Design review of the part built by this model. Coordinates are the model's own, in mm. A direction names the side the tool comes from. Round coordinates to 2 decimals unless told otherwise and drop trailing zeros. Order: outer loops, then holes, each group sorted by start corner. A loop starts at its lowest first (then second) coordinate and runs counter-clockwise, first axis right, second up. Notation, with made-up numbers: (67, 18) - (116, 18) arc R20 cw to (116, 36) - close; hole circle Ø7 at (22, 14). An arc over 180 degrees is marked (long way). Write item = value, one per line.
from build123d import *

# Parameters (mm, degrees)
SKETCH_3_W           = 2
SKETCH_3_H           = 46.5
SKETCH_4_W           = 1
SKETCH_4_H           = 47.5
SKETCH_5_W           = 2
SKETCH_5_H           = 46.5
SKETCH_6_R           = 9.5
CUT_EXTRUDE_1_DEPTH  = 328.171973127
SKETCH_7_R           = 9.5
CUT_EXTRUDE_2_DEPTH  = 328.171973127
SKETCH_8_R           = 9.5
CUT_EXTRUDE_3_DEPTH  = 328.171973127
SKETCH_9_R           = 9.5
CUT_EXTRUDE_4_DEPTH  = 328.171973127
SKETCH_10_R          = 9.5
CUT_EXTRUDE_5_DEPTH  = 328.171973127
SKETCH_11_R          = 9.5
CUT_EXTRUDE_6_DEPTH  = 328.171973127
SKETCH_12_R          = 9.5
CUT_EXTRUDE_7_DEPTH  = 328.171973127
SKETCH_13_R          = 9.5
CUT_EXTRUDE_8_DEPTH  = 328.171973127
SKETCH_14_R          = 9.5
CUT_EXTRUDE_9_DEPTH  = 328.171973127
SKETCH_15_R          = 9.5
CUT_EXTRUDE_10_DEPTH = 328.171973127
SKETCH_16_R          = 9.5
CUT_EXTRUDE_11_DEPTH = 328.171973127
SKETCH_17_R          = 9.5
CUT_EXTRUDE_12_DEPTH = 328.171973127


with BuildPart() as part:
    # Эскиз1 → Повернуть1 (revolve)
    with BuildSketch(Plane.XY, mode=Mode.PRIVATE) as revolve_1_sk:
        Polygon((0, 0), (273, 0), (273, 98.4), (271.4, 100), (265, 100), (265, 127.5), (247, 127.5), (247, 100), (239, 100), (239, 62.5), (215, 62.5), (215, 55), (183, 55), (178.669872981, 52.5), (95, 52.5), (95, 50), (42, 50), (42, 45), (0, 45), align=None)
    revolve(revolve_1_sk.sketch.rotate(Axis((0, 0, 0), (1, 0, 0)), 90), axis=Axis((0, 0, 0), (1, 0, 0)))

    # Эскиз2 → Вырез-Повернуть1 (revolve, cut)
    with BuildSketch(Plane.XY, mode=Mode.PRIVATE) as cut_revolve_1_sk:
        Polygon((0, 0), (273, 0), (273, 95), (265, 95), (265, 45), (254, 45), (254, 39), (240, 39), (240, 34), (203.5, 34), (203.5, 31), (0, 31), align=None)
    revolve(cut_revolve_1_sk.sketch.rotate(Axis((0, 0, 0), (1, 0, 0)), 90), axis=Axis((0, 0, 0), (1, 0, 0)), mode=Mode.SUBTRACT)

    # Эскиз3 → Rear_recess_left (revolve, cut)
    with BuildSketch(Plane.XY, mode=Mode.PRIVATE) as rear_recess_left_sk:
        with Locations((261, 71.75)):
            Rectangle(SKETCH_3_W, SKETCH_3_H)
    revolve(rear_recess_left_sk.sketch.rotate(Axis((0, 0, 0), (1, 0, 0)), 90), axis=Axis((0, 0, 0), (1, 0, 0)), mode=Mode.SUBTRACT)

    # Эскиз4 → Collar_groove_nominal (revolve, cut)
    with BuildSketch(Plane.XY, mode=Mode.PRIVATE) as collar_groove_nominal_sk:
        with Locations((262.5, 71.25)):
            Rectangle(SKETCH_4_W, SKETCH_4_H)
    revolve(collar_groove_nominal_sk.sketch.rotate(Axis((0, 0, 0), (1, 0, 0)), 90), axis=Axis((0, 0, 0), (1, 0, 0)), mode=Mode.SUBTRACT)

    # Эскиз5 → Rear_recess_lip (revolve, cut)
    with BuildSketch(Plane.XY, mode=Mode.PRIVATE) as rear_recess_lip_sk:
        with Locations((264, 71.75)):
            Rectangle(SKETCH_5_W, SKETCH_5_H)
    revolve(rear_recess_lip_sk.sketch.rotate(Axis((0, 0, 0), (1, 0, 0)), 90), axis=Axis((0, 0, 0), (1, 0, 0)), mode=Mode.SUBTRACT)

    # Эскиз6 → Вырез-Вытянуть1 (cut, through all)
    with BuildSketch(Plane(origin=(0, 0, 0), x_dir=(0, 0, -1), z_dir=(1, 0, 0))):
        with Locations(Location((0, 113, 0), (0, 0, 180))):
            Circle(SKETCH_6_R)
    extrude(amount=CUT_EXTRUDE_1_DEPTH, mode=Mode.SUBTRACT)

    # Эскиз7 → Вырез-Вытянуть2 (cut, through all)
    with BuildSketch(Plane(origin=(0, 0, 0), x_dir=(0, 0, -1), z_dir=(1, 0, 0))):
        with Locations(Location((-56.5, 97.860870628, 0), (0, 0, 180))):
            Circle(SKETCH_7_R)
    extrude(amount=CUT_EXTRUDE_2_DEPTH, mode=Mode.SUBTRACT)

    # Эскиз8 → Вырез-Вытянуть3 (cut, through all)
    with BuildSketch(Plane(origin=(0, 0, 0), x_dir=(0, 0, -1), z_dir=(1, 0, 0))):
        with Locations(Location((-97.860870628, 56.5, 0), (0, 0, 180))):
            Circle(SKETCH_8_R)
    extrude(amount=CUT_EXTRUDE_3_DEPTH, mode=Mode.SUBTRACT)

    # Эскиз9 → Вырез-Вытянуть4 (cut, through all)
    with BuildSketch(Plane(origin=(0, 0, 0), x_dir=(0, 0, -1), z_dir=(1, 0, 0))):
        with Locations(Location((-113, 0, 0), (0, 0, 180))):
            Circle(SKETCH_9_R)
    extrude(amount=CUT_EXTRUDE_4_DEPTH, mode=Mode.SUBTRACT)

    # Эскиз10 → Вырез-Вытянуть5 (cut, through all)
    with BuildSketch(Plane(origin=(0, 0, 0), x_dir=(0, 0, -1), z_dir=(1, 0, 0))):
        with Locations(Location((-97.860870628, -56.5, 0), (0, 0, 180))):
            Circle(SKETCH_10_R)
    extrude(amount=CUT_EXTRUDE_5_DEPTH, mode=Mode.SUBTRACT)

    # Эскиз11 → Вырез-Вытянуть6 (cut, through all)
    with BuildSketch(Plane(origin=(0, 0, 0), x_dir=(0, 0, -1), z_dir=(1, 0, 0))):
        with Locations(Location((-56.5, -97.860870628, 0), (0, 0, 180))):
            Circle(SKETCH_11_R)
    extrude(amount=CUT_EXTRUDE_6_DEPTH, mode=Mode.SUBTRACT)

    # Эскиз12 → Вырез-Вытянуть7 (cut, through all)
    with BuildSketch(Plane(origin=(0, 0, 0), x_dir=(0, 0, -1), z_dir=(1, 0, 0))):
        with Locations(Location((0, -113, 0), (0, 0, 180))):
            Circle(SKETCH_12_R)
    extrude(amount=CUT_EXTRUDE_7_DEPTH, mode=Mode.SUBTRACT)

    # Эскиз13 → Вырез-Вытянуть8 (cut, through all)
    with BuildSketch(Plane(origin=(0, 0, 0), x_dir=(0, 0, -1), z_dir=(1, 0, 0))):
        with Locations(Location((56.5, -97.860870628, 0), (0, 0, 180))):
            Circle(SKETCH_13_R)
    extrude(amount=CUT_EXTRUDE_8_DEPTH, mode=Mode.SUBTRACT)

    # Эскиз14 → Вырез-Вытянуть9 (cut, through all)
    with BuildSketch(Plane(origin=(0, 0, 0), x_dir=(0, 0, -1), z_dir=(1, 0, 0))):
        with Locations(Location((97.860870628, -56.5, 0), (0, 0, 180))):
            Circle(SKETCH_14_R)
    extrude(amount=CUT_EXTRUDE_9_DEPTH, mode=Mode.SUBTRACT)

    # Эскиз15 → Вырез-Вытянуть10 (cut, through all)
    with BuildSketch(Plane(origin=(0, 0, 0), x_dir=(0, 0, -1), z_dir=(1, 0, 0))):
        with Locations(Location((113, 0, 0), (0, 0, 180))):
            Circle(SKETCH_15_R)
    extrude(amount=CUT_EXTRUDE_10_DEPTH, mode=Mode.SUBTRACT)

    # Эскиз16 → Вырез-Вытянуть11 (cut, through all)
    with BuildSketch(Plane(origin=(0, 0, 0), x_dir=(0, 0, -1), z_dir=(1, 0, 0))):
        with Locations(Location((97.860870628, 56.5, 0), (0, 0, 180))):
            Circle(SKETCH_16_R)
    extrude(amount=CUT_EXTRUDE_11_DEPTH, mode=Mode.SUBTRACT)

    # Эскиз17 → Вырез-Вытянуть12 (cut, through all)
    with BuildSketch(Plane(origin=(0, 0, 0), x_dir=(0, 0, -1), z_dir=(1, 0, 0))):
        with Locations(Location((56.5, 97.860870628, 0), (0, 0, 180))):
            Circle(SKETCH_17_R)
    extrude(amount=CUT_EXTRUDE_12_DEPTH, mode=Mode.SUBTRACT)


solid = part.part
Item 1: Take a section at A-A, the plane z = -113. State the section outline as (x, y) points.
Data:
outline = (247, -59.05) - (265, -59.05) - (265, -9.5) - (247, -9.5) - close; (247, 9.5) - (265, 9.5) - (265, 59.05) - (247, 59.05) - close
Item 2: The part is to be moulded in two halves that separate along Z. For faces 6 (the face through (255.87, 103.58, -1.24)), 7 (the face through (255.874, -103.726, -2.059)), 8 (the face through (247, 66, -76)), 9 (the face through (198.776, 48.794, 25.379)), say which applies: +Z half, -Z half, draft (parallel to the pull), parting line (faces both ways), or undercut.
Data:
face_6 = undercut
face_7 = undercut
face_8 = draft
face_9 = parting line
Item 3: Take a section at C-C, the plane x = 74. State the section outline as (y, z) points.
Data:
outline = circle Ø100 at (0, 0); hole circle Ø62 at (0, 0)
Item 4: For line 1 along Y through (x, z) = (245, 0); line 2 along Y through (x, z) = (258, -51.5); line 3 along Y through (x, z) = (256, -56.5), list the stretches that pass through material, from the lowest coordinate up. Write a range as [from, to].
Data:
line_1 = [-100, -39], [39, 100]
line_2 = [-116.64, -105.94], [-89.78, 89.78], [105.94, 116.64]
line_3 = [-114.3, -107.36], [-88.36, 88.36], [107.36, 114.3]
Item 5: For faces 1 (the face through (262, 32, -36)), 2 (the face through (0, -10.6, 29.4)), 3 (the face through (255.874, 95.007, 65.561)), 4 (the face through (266.41, 92.74, -20.59)), 5 (the face through (242.94, -30.04, 95.38)), list the 3-axis set-ups (+Z, -Z, +X, -X, +Y, -Y) from which the entire face can be reached by the end or side of a thin tool; tool diameter is ignored.
Data:
face_1 = none
face_2 = +Z, -Z, -X, +Y, -Y
face_3 = +X, -X
face_4 = +X
face_5 = -X
Item 6: Insertion check: P1, Ø24.5, axis at y = -113, z = 0, coming from the -X side; P2, Ø24.5, axis at y = -97.86, z = 56.5, coming from the +X side; P3, Ø1, axis at x = 212, y = -44, coming from the +Z side. Each pin has a flat end and moves straight along its axis. Give the tip position at first contact, or say it passes through.
Data:
P1 = 247
P2 = 265
P3 = 33.66
